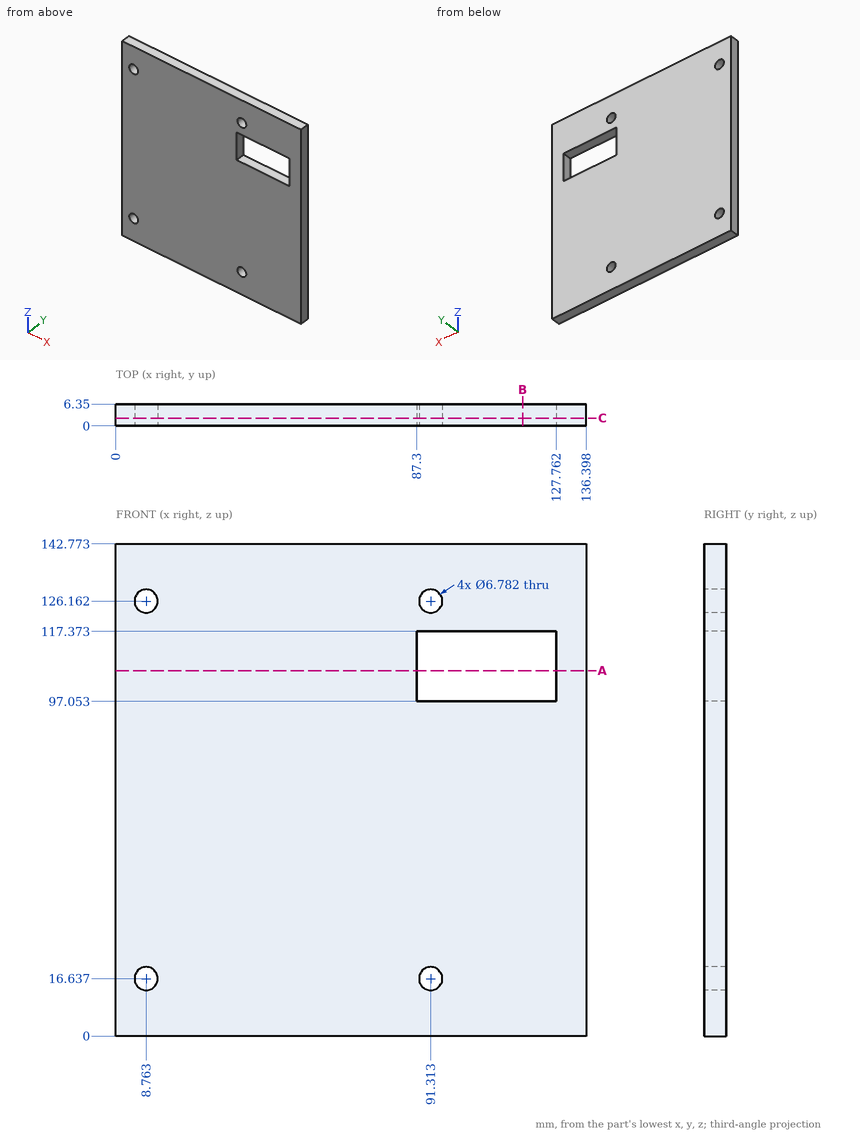
Geometry check sheet. Reference: drawing and pictorial views, mm from the part's lowest x, y, z. Coordinates: 2 decimals unless noted, no trailing zeros. Write each loop counter-clockwise with the first axis right and the second up, starting at its lowest first coordinate (ties: lowest second). Pieces come first, ordered by that corner, then holes.
Item 1: Cross-section at B-B on x = 118. Record the boundary of the cut face in (y, z).
Numbers:
outline: (0, 0) - (6.35, 0) - (6.35, 97.05) - (0, 97.05) - close; (0, 117.37) - (6.35, 117.37) - (6.35, 142.77) - (0, 142.77) - close
Item 2: Cross-section at A-A on z = 106. Record the boundary of the cut face in (x, y), then the cut area to 3 significant figures.
Numbers:
outline: (0, 0) - (87.3, 0) - (87.3, 6.35) - (0, 6.35) - close; (127.76, 0) - (136.4, 0) - (136.4, 6.35) - (127.76, 6.35) - close
area: 609 mm2
Item 3: Scan lines: probe 1 along Z at (x, y) = (105, 5.5); probe 2 along X at (y, z) = (2.5, 127); probe 3 along X at (y, z) = (2.25, 104.5). Record each from-to range of solid material in increasing order.
Numbers:
probe 1: z = 0 to 97.05, 117.37 to 142.77
probe 2: x = 0 to 5.48, 12.05 to 88.03, 94.6 to 136.4
probe 3: x = 0 to 87.3, 127.76 to 136.4
Item 4: Cross-section at C-C on y = 2.25. Record the boundary of the cut face in (x, z).
Numbers:
outline: (0, 0) - (136.4, 0) - (136.4, 142.77) - (0, 142.77) - close; hole circle Ø6.78 at (8.76, 16.64); hole circle Ø6.78 at (8.76, 126.16); hole (87.3, 97.05) - (127.76, 97.05) - (127.76, 117.37) - (87.3, 117.37) - close; hole circle Ø6.78 at (91.31, 16.64); hole circle Ø6.78 at (91.31, 126.16)
